```python
from build123d import *

# Parameters (mm, degrees)
SKETCH1_R           = 2.6
BOSS_EXTRUDE1_DEPTH = 3
SKETCH2_W           = 3
SKETCH2_H           = 3.2
SKETCH2_W_2         = 19
SKETCH2_R           = 1.6
CUT_EXTRUDE1_DEPTH  = 10
FILLET1_R           = 5
SKETCH3_R           = 1.6
CUT_EXTRUDE2_DEPTH  = 321.989096388
SKETCH4_W           = 47.2
SKETCH4_H           = 5.5
SKETCH4_W_2         = 3
CUT_EXTRUDE3_DEPTH  = 321.989096388
FILLET2_R           = 5


with BuildPart() as part:
    # Sketch1 → Boss-Extrude1 (new body)
    # profile 1 of 2: a face of its own
    with BuildSketch(Plane(origin=(0, 0, 0), x_dir=(1, 0, 0), z_dir=(0, 1, 0))):
        with BuildLine():
            Line((0, -45), (260, -45))
            ThreePointArc((260, -45), (305, 0), (260, 45))
            Line((260, 45), (0, 45))
            ThreePointArc((0, 45), (-45, 0), (0, -45))
        make_face()
        with Locations(Location((0, 0, 0), (0, 0, 270))):
            Circle(SKETCH1_R, mode=Mode.SUBTRACT)
        with BuildLine():
            ThreePointArc((250, 2.6), (247.4, 0), (250, -2.6))
            Line((250, -2.6), (270, -2.6))
            ThreePointArc((270, -2.6), (272.6, 0), (270, 2.6))
            Line((270, 2.6), (250, 2.6))
        make_face(mode=Mode.SUBTRACT)
    # profile 2 of 2: a face of its own
    with BuildSketch(Plane(origin=(0, 0, 0), x_dir=(1, 0, 0), z_dir=(0, 1, 0))):
        with BuildLine():
            ThreePointArc((-45, 0), (-31.819805153, 31.819805153), (0, 45))
            Line((0, 45), (260, 45))
            ThreePointArc((260, 45), (291.819805153, 31.819805153), (305, 0))
            Line((305, 0), (305, 100))
            Line((305, 100), (-45, 100))
            Line((-45, 100), (-45, 0))
        make_face()
    extrude(amount=BOSS_EXTRUDE1_DEPTH)

    # Sketch2 → Cut-Extrude1 (cut)
    with BuildSketch(Plane.XZ):
        with Locations((81.5, -35)):
            Rectangle(SKETCH2_W, SKETCH2_H)
        with BuildLine():
            Line((80, -33.4), (83, -33.4))
            ThreePointArc((83, -33.4), (81.5, -31.9), (80, -33.4))
        make_face()
        with BuildLine():
            ThreePointArc((80, -36.6), (81.5, -38.1), (83, -36.6))
            Line((83, -36.6), (80, -36.6))
        make_face()
        with Locations((92.5, -35)):
            Rectangle(SKETCH2_W_2, SKETCH2_H)
        with BuildLine():
            ThreePointArc((105, -33.4), (103.5, -31.9), (102, -33.4))
            Line((102, -33.4), (105, -33.4))
        make_face()
        with Locations((103.5, -35)):
            Rectangle(SKETCH2_W, SKETCH2_H)
        with BuildLine():
            Line((105, -36.6), (102, -36.6))
            ThreePointArc((102, -36.6), (103.5, -38.1), (105, -36.6))
        make_face()
        with BuildLine():
            ThreePointArc((83, -73.4), (81.5, -71.9), (80, -73.4))
            Line((80, -73.4), (83, -73.4))
        make_face()
        with Locations((81.5, -75)):
            Rectangle(SKETCH2_W, SKETCH2_H)
        with Locations((92.5, -75)):
            Rectangle(SKETCH2_W_2, SKETCH2_H)
        with BuildLine():
            Line((83, -76.6), (80, -76.6))
            ThreePointArc((80, -76.6), (81.5, -78.1), (83, -76.6))
        make_face()
        with BuildLine():
            ThreePointArc((105, -73.4), (103.5, -71.9), (102, -73.4))
            Line((102, -73.4), (105, -73.4))
        make_face()
        with Locations((103.5, -75)):
            Rectangle(SKETCH2_W, SKETCH2_H)
        with BuildLine():
            Line((105, -76.6), (102, -76.6))
            ThreePointArc((102, -76.6), (103.5, -78.1), (105, -76.6))
        make_face()
        with BuildLine():
            Line((155, -33.4), (158, -33.4))
            ThreePointArc((158, -33.4), (156.5, -31.9), (155, -33.4))
        make_face()
        with Locations((156.5, -35)):
            Rectangle(SKETCH2_W, SKETCH2_H)
        with BuildLine():
            ThreePointArc((155, -36.6), (156.5, -38.1), (158, -36.6))
            Line((158, -36.6), (155, -36.6))
        make_face()
        with Locations((167.5, -35)):
            Rectangle(SKETCH2_W_2, SKETCH2_H)
        with BuildLine():
            Line((177, -33.4), (180, -33.4))
            ThreePointArc((180, -33.4), (178.5, -31.9), (177, -33.4))
        make_face()
        with Locations((178.5, -35)):
            Rectangle(SKETCH2_W, SKETCH2_H)
        with BuildLine():
            ThreePointArc((177, -36.6), (178.5, -38.1), (180, -36.6))
            Line((180, -36.6), (177, -36.6))
        make_face()
        with BuildLine():
            ThreePointArc((158, -73.4), (156.5, -71.9), (155, -73.4))
            Line((155, -73.4), (158, -73.4))
        make_face()
        with Locations((156.5, -75)):
            Rectangle(SKETCH2_W, SKETCH2_H)
        with BuildLine():
            Line((158, -76.6), (155, -76.6))
            ThreePointArc((155, -76.6), (156.5, -78.1), (158, -76.6))
        make_face()
        with Locations((167.5, -75)):
            Rectangle(SKETCH2_W_2, SKETCH2_H)
        with BuildLine():
            ThreePointArc((180, -73.4), (178.5, -71.9), (177, -73.4))
            Line((177, -73.4), (180, -73.4))
        make_face()
        with Locations((178.5, -75)):
            Rectangle(SKETCH2_W, SKETCH2_H)
        with BuildLine():
            Line((180, -76.6), (177, -76.6))
            ThreePointArc((177, -76.6), (178.5, -78.1), (180, -76.6))
        make_face()
        with Locations(Location((200, -75, 0), (0, 0, 270))):
            Circle(SKETCH2_R)
        with Locations(Location((290, -92, 0), (0, 0, 270))):
            Circle(SKETCH2_R)
        with Locations(Location((270, -92, 0), (0, 0, 270))):
            Circle(SKETCH2_R)
        with Locations(Location((60, -35, 0), (0, 0, 90))):
            Circle(SKETCH2_R)
        with Locations(Location((60, -75, 0), (0, 0, 270))):
            Circle(SKETCH2_R)
        with Locations(Location((-10, -92, 0), (0, 0, 270))):
            Circle(SKETCH2_R)
        with Locations(Location((-30, -92, 0), (0, 0, 270))):
            Circle(SKETCH2_R)
        with Locations(Location((200, -35, 0), (0, 0, 270))):
            Circle(SKETCH2_R)
    extrude(amount=-CUT_EXTRUDE1_DEPTH, mode=Mode.SUBTRACT)

    # Fillet1
    fillet1_edges = [part.edges().sort_by_distance(p)[0] for p in [
        (-45, 1.5, -100),
        (305, 1.5, -100),
    ]]
    fillet(fillet1_edges, radius=FILLET1_R)

    # Sketch3 → Cut-Extrude2 (cut, through all)
    with BuildSketch(Plane.XZ):
        with Locations(Location((105, 35, 0), (0, 0, 270))):
            Circle(SKETCH3_R)
        with Locations(Location((155, 35, 0), (0, 0, 270))):
            Circle(SKETCH3_R)
        with BuildLine():
            Line((193.4, -1.6), (153.4, -1.6))
            ThreePointArc((153.4, -1.6), (151.8, 0), (153.4, 1.6))
            Line((153.4, 1.6), (193.4, 1.6))
            ThreePointArc((193.4, 1.6), (195, 0), (193.4, -1.6))
        make_face()
    extrude(amount=-CUT_EXTRUDE2_DEPTH, mode=Mode.SUBTRACT)

    # Sketch4 → Cut-Extrude3 (cut, through all)
    with BuildSketch(Plane(origin=(0, 3, 0), x_dir=(1, 0, 0), z_dir=(0, 1, 0))):
        with Locations((-21.4, 81.25)):
            Rectangle(SKETCH4_W, SKETCH4_H)
        with Locations((3.7, 81.25)):
            Rectangle(SKETCH4_W_2, SKETCH4_H)
        with BuildLine():
            ThreePointArc((5.2, 84), (3.7, 85.5), (2.2, 84))
            Line((2.2, 84), (5.2, 84))
        make_face()
        with BuildLine():
            Line((5.2, 78.5), (2.2, 78.5))
            ThreePointArc((2.2, 78.5), (3.7, 77), (5.2, 78.5))
        make_face()
        with BuildLine():
            ThreePointArc((257.8, 84), (256.3, 85.5), (254.8, 84))
            Line((254.8, 84), (257.8, 84))
        make_face()
        with Locations((256.3, 81.25)):
            Rectangle(SKETCH4_W_2, SKETCH4_H)
        with BuildLine():
            Line((257.8, 78.5), (254.8, 78.5))
            ThreePointArc((254.8, 78.5), (256.3, 77), (257.8, 78.5))
        make_face()
        with Locations((281.4, 81.25)):
            Rectangle(SKETCH4_W, SKETCH4_H)
    extrude(amount=-CUT_EXTRUDE3_DEPTH, mode=Mode.SUBTRACT)

    # Fillet2
    fillet2_edges = [part.edges().sort_by_distance(p)[0] for p in [
        (-45, 1.5, -78.5),
        (-45, 1.5, -84),
        (305, 1.5, -84),
        (305, 1.5, -78.5),
    ]]
    fillet(fillet2_edges, radius=FILLET2_R)


solid = part.part
```
The model under review builds one solid part; all positions refer to its coordinate system, in mm. Give positions to 0.01 mm unless a question says otherwise; leave off trailing zeros. Write each loop counter-clockwise with the first axis right and the second up, starting at its lowest first coordinate (ties: lowest second). Pieces come first, ordered by that corner, then holes.
(1) Consider section A-A, the plane x = 91. Give the boundary of the cut face in (y, z).
(2) Consider section B-B, the plane y = 0.65. Give the number of separate pieces and of enclosed holes in the cut face, and give its area (3 significant figures).
(3) Consider section C-C, the plane x = 278. Give the boundary of the cut face in (y, z).
(4) Consider section D-D, the plane z = 20.5. Give the boundary of the cut face in (x, y), and give its area (3 significant figures).
(5) To check wall thickness, follow L1, parallel to Z at x = 170, y = 1.4; L2, parallel to X at y = 1.5, z = -92; L3, parallel to Z at x = 258, y = 2.7. State the ranges of each line that lie inside material, in increasing order.
(6) For P1, Ø3, axis at x = 155, z = 35, coming from the -Y side, flat-tipped, find the tip position at first contact; note if it passes through.
Returned:
1. outline: (0, -100) - (3, -100) - (3, -76.6) - (0, -76.6) - close; (0, -73.4) - (3, -73.4) - (3, -36.6) - (0, -36.6) - close; (0, -33.4) - (3, -33.4) - (3, 45) - (0, 45) - close
2. separate pieces: 1
2. enclosed holes: 17
2. area: 48,500 mm2
3. outline: (0, -100) - (3, -100) - (3, -84) - (0, -84) - close; (0, -78.5) - (3, -78.5) - (3, 41.24) - (0, 41.24) - close
4. outline: (-40.06, 0) - (300.06, 0) - (300.06, 3) - (-40.06, 3) - close
4. area: 1,020 mm2
5. L1: z = -100 to -76.6, -73.4 to -36.6, -33.4 to -1.6, 1.6 to 45
5. L2: x = -45 to -31.6, -28.4 to -11.6, -8.4 to 268.4, 271.6 to 288.4, 291.6 to 305
5. L3: z = -100 to -84, -78.5 to -2.6, 2.6 to 45
6. P1: passes through
